Source: CAD feature listing. Evaluate the final solid. Frame: model axes, mm. A direction names the side the tool comes from. Give positions to 0.01 mm unless a question says otherwise; leave off trailing zeros. Loops run counter-clockwise (first coordinate to the right, second up) from the corner with the lowest first, then second, coordinate; pieces in that order, holes last. Notation, with made-up numbers: M -19.5,11 L -8.5,11 A14 cw -8.5,21 Z; hole C 24,-11.5 d7. An arc over 180 degrees is marked long. Put each result on its own line as item: value. Start each with the question number.
```python
from build123d import *

# Parameters (mm, degrees)
SKETCH1_R           = 50
SKETCH1_R_2         = 18
SKETCH1_R_3         = 5
BOSS_EXTRUDE1_DEPTH = 20
CUT_EXTRUDE1_START  = -8
SKETCH2_R           = 31
SKETCH2_R_2         = 18
CUT_EXTRUDE1_DEPTH  = 8


with BuildPart() as part:
    # Sketch1 → Boss-Extrude1 (new body)
    with BuildSketch(Plane.XY):
        Circle(SKETCH1_R)
        Circle(SKETCH1_R_2, mode=Mode.SUBTRACT)
        with Locations((0, -41)):
            Circle(SKETCH1_R_3, mode=Mode.SUBTRACT)
        with Locations((-24.099195344, -33.169696769)):
            Circle(SKETCH1_R_3, mode=Mode.SUBTRACT)
        with Locations((-38.993317168, -12.669696769)):
            Circle(SKETCH1_R_3, mode=Mode.SUBTRACT)
        with Locations((-38.993317168, 12.669696769)):
            Circle(SKETCH1_R_3, mode=Mode.SUBTRACT)
        with Locations((-24.099195344, 33.169696769)):
            Circle(SKETCH1_R_3, mode=Mode.SUBTRACT)
        with Locations((0, 41)):
            Circle(SKETCH1_R_3, mode=Mode.SUBTRACT)
        with Locations((24.099195344, 33.169696769)):
            Circle(SKETCH1_R_3, mode=Mode.SUBTRACT)
        with Locations((38.993317168, 12.669696769)):
            Circle(SKETCH1_R_3, mode=Mode.SUBTRACT)
        with Locations((38.993317168, -12.669696769)):
            Circle(SKETCH1_R_3, mode=Mode.SUBTRACT)
        with Locations((24.099195344, -33.169696769)):
            Circle(SKETCH1_R_3, mode=Mode.SUBTRACT)
    extrude(amount=BOSS_EXTRUDE1_DEPTH)

    # Sketch2 → Cut-Extrude1 (cut)
    with BuildSketch(Plane.XY.offset(20).offset(CUT_EXTRUDE1_START)):
        Circle(SKETCH2_R)
        Circle(SKETCH2_R_2, mode=Mode.SUBTRACT)
    extrude(amount=CUT_EXTRUDE1_DEPTH, mode=Mode.SUBTRACT)


solid = part.part
```
1. Section C-C, the plane x = -25. Output: boundary loops of the cut face in (y, z).
2. Ray query, line 1 (Y direction, x = 23, z = 14); line 2 (Y direction, x = 37.5, z = 4.25); line 3 (Y direction, x = 23.5, z = 17.5). Return the intervals inside material, ascending.
3. Set-up query: faces 1 (the face through (-4.036, 30.736, 15.944)), 2 (the face through (3, -37, 10)). Return all of +Z, -Z, +X, -X, +Y, -Y with unobstructed straight access to the full face (end or side cutting, diameter ignored); none if empty.
4. Section B-B, the plane y = 0. Output: boundary loops of the cut face in (x, z).
5. Pull-direction query (Y, two-part tool) for faces 3 (the face through (-1, -22, 0)), 4 (the face through (34, 12.9, 9.9)), 5 (the face through (47.69, 15.02, 9.86)); classes: released by +Y, released by -Y, zero draft, split by the parting line, or undercut.
6. Contact query for flat-ended pins moving along their axis: pin 1 (8 mm diameter, centred on x = 0, y = -41, fed in from +Z); pin 2 (10 mm diameter, centred on y = 34.5, z = 3, fed in from +X); pin 3 (6 mm diameter, centred on y = -37, z = 3.5, fed in from -X); pin 4 (10 mm diameter, centred on x = -22, z = 8.5, fed in from +Y). Output: stop coordinate, or through.
7. Section A-A, the plane x = 0. Output: boundary loops of the cut face in (y, z).
8. Section D-D, the plane z = 2.5. State how many separate pieces and enclosed holes the cut face has, plus the area to 3 significant figures.
Results found:
1. outline: M -43.3,0 L -38.09,0 L -38.09,20 L -43.3,20 Z; M -28.25,0 L 28.25,0 L 28.25,20 L 18.33,20 L 18.33,12 L -18.33,12 L -18.33,20 L -28.25,20 Z; M 38.09,0 L 43.3,0 L 43.3,20 L 38.09,20 Z
2. line 1: -44.4 to -38.05, -28.29 to -20.78, 20.78 to 28.29, 38.05 to 44.4
2. line 2: -33.07 to -17.44, -7.9 to 7.9, 17.44 to 33.07
2. line 3: -44.13 to -38.13, -28.21 to -20.22, 20.22 to 28.21, 38.13 to 44.13
3. face 1: +Z
3. face 2: +Z, -Z
4. outline: M -50,0 L -18,0 L -18,12 L -31,12 L -31,20 L -50,20 Z; M 18,0 L 50,0 L 50,20 L 31,20 L 31,12 L 18,12 Z
5. face 3: zero draft
5. face 4: undercut
5. face 5: split by the parting line
6. pin 1: through
6. pin 2: x = 40.37
6. pin 3: x = -36.66
6. pin 4: y = 47.02
7. outline: M -50,0 L -46,0 L -46,20 L -50,20 Z; M -36,0 L -18,0 L -18,12 L -31,12 L -31,20 L -36,20 Z; M 18,0 L 36,0 L 36,20 L 31,20 L 31,12 L 18,12 Z; M 46,0 L 50,0 L 50,20 L 46,20 Z
8. separate pieces: 1
8. enclosed holes: 11
8. area: 6,050 mm²
